```python
from build123d import *

# Parameters (mm, degrees)
F0_R     = 53.975
F1_DEPTH = 19.05
F2_R     = 29.87
F2_R_2   = 9.55
F3_DEPTH = 29.21
F5_D     = 6.7564
F6_R     = 53.975
F6_R_2   = 37.846
F7_DEPTH = 7.62
F8_R     = 9.525
F9_DEPTH = 55.881
F10_R    = 7.62


with BuildPart() as f1:
    # F0 (on Top) → F1 (new body)
    with BuildSketch(Plane.XY):
        Circle(F0_R)
    extrude(amount=F1_DEPTH)

    # F2 (on face) → F3 (join)
    with BuildSketch(Plane.XY.offset(19.05)):
        Circle(F2_R)
        Circle(F2_R_2, mode=Mode.SUBTRACT)
    extrude(amount=F3_DEPTH)

    # F5 (through all)
    with Locations(Plane.XY.offset(48.26)):
        with Locations((-22.25, 0), (0, 22.25), (22.25, 0), (0, -22.25)):
            Hole(F5_D / 2)

    # F6 (on face) → F7 (join)
    with BuildSketch(Plane(origin=(0, 0, 0), x_dir=(1, 0, 0), z_dir=(0, 0, -1))):
        Circle(F6_R)
        Circle(F6_R_2, mode=Mode.SUBTRACT)
    extrude(amount=F7_DEPTH)

    # F8 (on face) → F9 (cut, through all)
    with BuildSketch(Plane.XY.offset(48.26)):
        with Locations((18.8585378542, -18.8585378542)):
            Circle(F8_R)
    extrude(amount=-F9_DEPTH, mode=Mode.SUBTRACT)

    # F10
    f10_edges = [f1.edges().sort_by_distance(p)[0] for p in [
        (26.682506, -13.426122, 33.655),
        (13.426122, -26.682506, 33.655),
    ]]
    fillet(f10_edges, radius=F10_R)


solid = f1.part
```
Could you check a few things on this model? Use its own coordinates, in mm. A direction names the side the tool comes from. Give positions to 0.01 mm unless a question says otherwise; leave off trailing zeros. Write each loop counter-clockwise with the first axis right and the second up, starting at its lowest first coordinate (ties: lowest second). Pieces come first, ordered by that corner, then holes. Notation, with made-up numbers: (87.5, 19.5) - (120.5, 19.5) arc R31 cw to (120.5, 53.5) - close; hole circle Ø5 at (10.5, -17.75). An arc over 180 degrees is marked (long way). One line per item, written item: value. Start each with the question number.
Item 1: I'm going to push flat-ended pins straight in: pin 1 (8 mm diameter, centred on x = 22.25, y = 0, fed in from +Z); pin 2 (1 mm diameter, centred on x = -37.5, z = 12.5, fed in from +Y); pin 3 (4 mm diameter, centred on x = 0, y = 22.25, fed in from +Z); pin 4 (1.5 mm diameter, centred on y = 22, z = 41.5, fed in from +X). Where does each tip first touch, or does it pass through?
Item 2: Imagine slicing it at D-D, the plane y = 32. List the corners of the cut face in (x, z) for me.
Item 3: Which directions (+Z, -Z, +X, -X, +Y, -Y) give clear straight access to the entire face, cutting with the end or side of a thin tool? Please do faces 4 (the face through (0, 0, 19.05)), 5 (the face through (-1, 1, 0)), 6 (the face through (0.44, -18.9, 23.79)).
Item 4: Imagine slicing it at A-A, the plane x = 0. List the corners of the cut face in (y, z) for me (3 decimals).
Item 5: If we mould it in two halves opening along Y, with no side actions, what happens to faces 1 (the face through (-39.78, -36.48, 5.9)), 2 (the face through (-7, 7, 48.26)), 3 (the face through (-7.58, -5.81, 33.45))? For each: +Y half, -Y half, draft (parallel to the pull), parting line (faces both ways), or undercut.
Item 6: Please list where these lines run through material, in increasing order: line 1 (Y direction, x = 0, z = 19.5); line 2 (Y direction, x = 0, z = 19) (3 decimals); line 3 (X direction, y = 0.5, z = 7). Write a range as from..to.
Item 7: Imagine slicing it at C-C, the plane x = 15. List the corners of the cut face in (y, z) for me.
Item 8: Imagine slicing it at B-B, the plane y = -16.5. List the corners of the cut face in (x, z) for me.
Geometry says:
1. pin 1: z = 48.26
1. pin 2: y = 39.3
1. pin 3: through
1. pin 4: x = 20.99
2. outline: (-43.47, -7.62) - (-20.21, -7.62) - (-20.21, 0) - (20.21, 0) - (20.21, -7.62) - (43.47, -7.62) - (43.47, 19.05) - (-43.47, 19.05) - close
3. face 4: +Z
3. face 5: -Z
3. face 6: +Z, -Z
4. outline: (-53.975, -7.62) - (-37.846, -7.62) - (-37.846, 0) - (-25.628, 0) - (-25.628, 48.26) - (-29.87, 48.26) - (-29.87, 19.05) - (-53.975, 19.05) - close; (-18.872, 0) - (18.872, 0) - (18.872, 48.26) - (9.55, 48.26) - (9.55, 19.05) - (-9.55, 19.05) - (-9.55, 48.26) - (-18.872, 48.26) - close; (25.628, 0) - (37.846, 0) - (37.846, -7.62) - (53.975, -7.62) - (53.975, 19.05) - (29.87, 19.05) - (29.87, 48.26) - (25.628, 48.26) - close
5. face 1: parting line
5. face 2: draft
5. face 3: undercut
6. line 1: -29.87..-25.63, -18.87..-9.55, 9.55..18.87, 25.63..29.87
6. line 2: -53.975..-25.628, -18.872..18.872, 25.628..53.975
6. line 3: -53.97..-25.59, -18.91..18.91, 25.59..53.97
7. outline: (-51.85, -7.62) - (-34.75, -7.62) - (-34.75, 0) - (-27.57, 0) - (-27.57, 19.05) - (-51.85, 19.05) - close; (-10.15, 0) - (34.75, 0) - (34.75, -7.62) - (51.85, -7.62) - (51.85, 19.05) - (25.83, 19.05) - (25.83, 48.26) - (-10.15, 48.26) - close
8. outline: (-51.39, -7.62) - (-34.06, -7.62) - (-34.06, 0) - (9.63, 0) - (9.63, 48.26) - (-24.9, 48.26) - (-24.9, 19.05) - (-51.39, 19.05) - close; (28.09, 0) - (34.06, 0) - (34.06, -7.62) - (51.39, -7.62) - (51.39, 19.05) - (28.09, 19.05) - close
